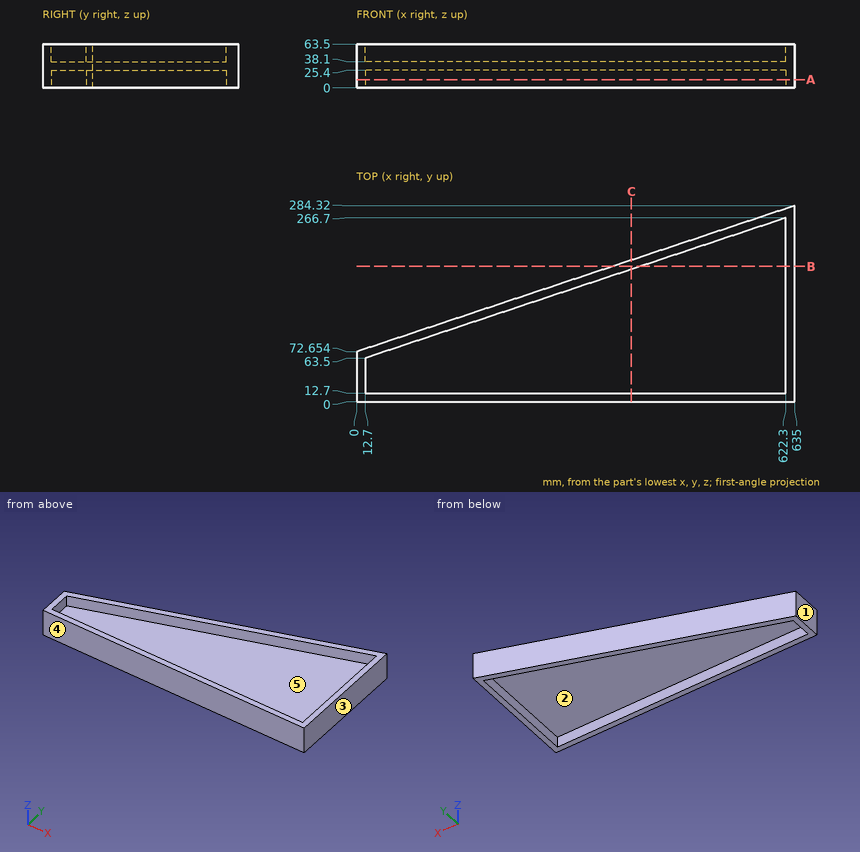
Part print with two shaded views. Sizes in mm from the minimum x, y, z corner. A direction names the side the tool comes from. Round coordinates to 2 decimals unless told otherwise and drop trailing zeros. Loops run counter-clockwise (first coordinate to the right, second up) from the corner with the lowest first, then second, coordinate; pieces in that order, holes last. Notation, with made-up numbers: (-33.5, 74.25) - (-5.5, 74.25) arc R26 ccw to (-5.5, 99.25) - close; hole circle Ø10 at (62, 75). An arc over 180 degrees is marked (long way). Answer as a JSON object with one key per item and string values.
Item 1: Band-saw the part on A-A on z = 12. List the corners of the cut face in (x, y).
Output:
{"outline": "(0, 0) - (635, 0) - (635, 284.32) - (0, 72.65) - close; hole (12.7, 12.7) - (622.3, 12.7) - (622.3, 266.7) - (12.7, 63.5) - close"}
Item 2: Pull direction X, two halves, no side cores. Call the marked faces 1, 2 and 3: pulls with the +X half, pulls with the -X half, needs draft (parallel to the pull), parting line crosses it, or undercut.
Output:
{"face 1": "pulls with the -X half", "face 2": "undercut", "face 3": "pulls with the +X half"}
Item 3: Band-saw the part on C-C on x = 398.5. List the corners of the cut face in (y, z).
Output:
{"outline": "(0, 0) - (12.7, 0) - (12.7, 25.4) - (192.1, 25.4) - (192.1, 0) - (205.49, 0) - (205.49, 63.5) - (192.1, 63.5) - (192.1, 38.1) - (12.7, 38.1) - (12.7, 63.5) - (0, 63.5) - close"}
Item 4: Tool access for the marked faces 4 and 5: list every direction of +Z, -Z, +X, -X, +Y, -Y with a clear straight run to the whole face (end or side of a thin tool).
Output:
{"face 4": "+Z, -Z, +X, -X, -Y", "face 5": "+Z"}
Item 5: Wall check: L1, parallel to Y at x = 45, z = 17; L2, parallel to Y at x = 394.5, z = 14; L3, parallel to Z at x = 70.5, y = 16. Give the ranges that are in metal, low to high.
Output:
{"L1": "0 to 12.7, 74.27 to 87.65", "L2": "0 to 12.7, 190.77 to 204.15", "L3": "25.4 to 38.1"}
Item 6: Pin check, flat tips, straight feed: pin 1 (12.5 mm diameter, centred on x = 308.5, z = 51, fed in from +Y); pin 2 (12 mm diameter, centred on x = 456, y = 166, fed in from -Z); pin 3 (20.5 mm diameter, centred on x = 296.5, z = 12.5, fed in from +Y). Stop position of each tip, or through.
Output:
{"pin 1": "y = 177.57", "pin 2": "z = 25.4", "pin 3": "y = 174.9"}
Item 7: Band-saw the part on B-B on y = 196.5. List the corners of the cut face in (x, z), plus the area to 3 significant figures.
Output:
{"outline": "(371.54, 0) - (411.7, 0) - (411.7, 25.4) - (622.3, 25.4) - (622.3, 0) - (635, 0) - (635, 63.5) - (622.3, 63.5) - (622.3, 38.1) - (411.7, 38.1) - (411.7, 63.5) - (371.54, 63.5) - close", "area": "6,030 mm2"}
